Check sheet for the modelled part. Datum: model origin and axes. Units: mm. A direction names the side the tool comes from. Round coordinates to 2 decimals unless told otherwise and drop trailing zeros. Loops run counter-clockwise (first coordinate to the right, second up) from the corner with the lowest first, then second, coordinate; pieces in that order, holes last. Notation, with made-up numbers: (14, 80) - (25, 80) arc R21 cw to (25, 105) - close; hole circle Ø8 at (56.5, 60). An arc over 180 degrees is marked (long way). Put each result on its own line as item: value. Start each with the question number.
```python
from build123d import *

# Parameters (mm, degrees)
F1_DEPTH = 31.75
F2_W     = 12.7
F2_H     = 50.8
F3_DEPTH = 12.7
F4_W     = 12.7
F4_H     = 50.8
F5_DEPTH = 12.7


with BuildPart() as f1:
    # F0 (on Front) → F1 (new body)
    with BuildSketch(Plane.XZ):
        Polygon((146.225058, 99.415574), (-218.899942, 99.415574), (-218.899942, -91.084426), (95.425058, -91.084426), (95.425058, 48.615574), (146.225058, 48.615574), align=None)
    extrude(amount=F1_DEPTH)

    # F2 (on face) → F3 (join)
    with BuildSketch(Plane.YZ.offset(146.225058)):
        with Locations((-15.875, 74.015574)):
            Rectangle(F2_W, F2_H)
    extrude(amount=F3_DEPTH)

    # F4 (on face) → F5 (join)
    with BuildSketch(Plane(origin=(-218.899942, 0, 0), x_dir=(0, -1, 0), z_dir=(-1, 0, 0))):
        with Locations((15.875, 74.015574)):
            Rectangle(F4_W, F4_H)
    extrude(amount=F5_DEPTH)


solid = f1.part
```
Q1. Cross-section at D-D on z = -72. Enter the section's corners in (x, y).
Q2. Set-up check for faces 1 (the face through (-225, -9.525, 74)), 2 (the face through (-225, -16, 48.616)), 3 (the face through (152, -9.525, 74)), 4 (the face through (152, -22.225, 74)): record each of +Z, -Z, +X, -X, +Y, -Y from which the full face is reachable in a straight line by a thin tool's end or side.
Q3. Depth check by flat-ended pin: pin 1 Ø2 at (y, z) = (-7, -9) entering from -X; pin 2 Ø7.5 at (y, z) = (-6.5, 76.5) entering from +X; pin 3 Ø6.5 at (x, y) = (-224.5, -18.5) entering from -Z; pin 4 Ø3 at (y, z) = (-11, 9) entering from +X. Enter the tip coordinate at first touch or a pass-through.
Q4. Cross-section at A-A on z = 82. Enter the section's corners in (x, y) (3 decimals), and give its area (3 significant figures).
Q5. Material ranges on line 1 (Z direction, x = 111, y = -5); line 2 (X direction, y = -2, z = -31), recorded low to high. Write a range as from..to.
Q6. Cross-section at B-B on y = -15. Enter the section's corners in (x, z), and give its area (4 significant figures).
Q7. Cross-section at C-C on x = 121. Enter the section's corners in (y, z).
Answer list:
1. outline: (-218.9, -31.75) - (95.43, -31.75) - (95.43, 0) - (-218.9, 0) - close
2. face 1: +Z, -Z, -X, +Y
2. face 2: -Z, -X, +Y, -Y
2. face 3: +Z, -Z, +X, +Y
2. face 4: +Z, -Z, +X, -Y
3. pin 1: stops at x = -218.9
3. pin 2: stops at x = 158.93
3. pin 3: stops at z = 48.62
3. pin 4: stops at x = 95.43
4. outline: (-231.6, -22.225) - (-218.9, -22.225) - (-218.9, -31.75) - (146.225, -31.75) - (146.225, -22.225) - (158.925, -22.225) - (158.925, -9.525) - (146.225, -9.525) - (146.225, 0) - (-218.9, 0) - (-218.9, -9.525) - (-231.6, -9.525) - close
4. area: 11,900 mm2
5. line 1: z = 48.62..99.42
5. line 2: x = -218.9..95.43
6. outline: (-231.6, 48.62) - (-218.9, 48.62) - (-218.9, -91.08) - (95.43, -91.08) - (95.43, 48.62) - (158.93, 48.62) - (158.93, 99.42) - (-231.6, 99.42) - close
6. area: 63,750 mm2
7. outline: (-31.75, 48.62) - (0, 48.62) - (0, 99.42) - (-31.75, 99.42) - close
